Verification items for this drawing (mm, ordinates from the low corner). Round coordinates to 2 decimals unless told otherwise and drop trailing zeros. Order: outer loops, then holes, each group sorted by start corner. A loop starts at its lowest first (then second) coordinate and runs counter-clockwise, first axis right, second up. Notation, with made-up numbers: (-34.75, 40) -> (-5.75, 40) arc R23 ccw to (-5.75, 48) -> close; hole circle Ø10 at (28.25, -11). An arc over 180 degrees is marked (long way). Answer in a Markdown table with one row per item. Add a question column.
1. Sectioned sample at B-B, the plane z = 10. Record the boundary of the cut face in (x, y), then the cut area to 3 significant figures.
2. Depth check by flat-ended pin: P1, Ø4.5, axis at x = 60, z = 60, coming from the +Y side. Enter the tip coordinate at first touch or a pass-through.
3. Sectioned sample at A-A, the plane x = 60. Record the boundary of the cut face in (y, z).
4. Material ranges on L1, parallel to Z at x = 60, y = 6; L2, parallel to X at y = 3.5, z = 59; L3, parallel to Z at x = 9.5, y = 1, recorded low to high. Write a range as from..to.
5. Sectioned sample at C-C, the plane y = 7. Record the boundary of the cut face in (x, z).
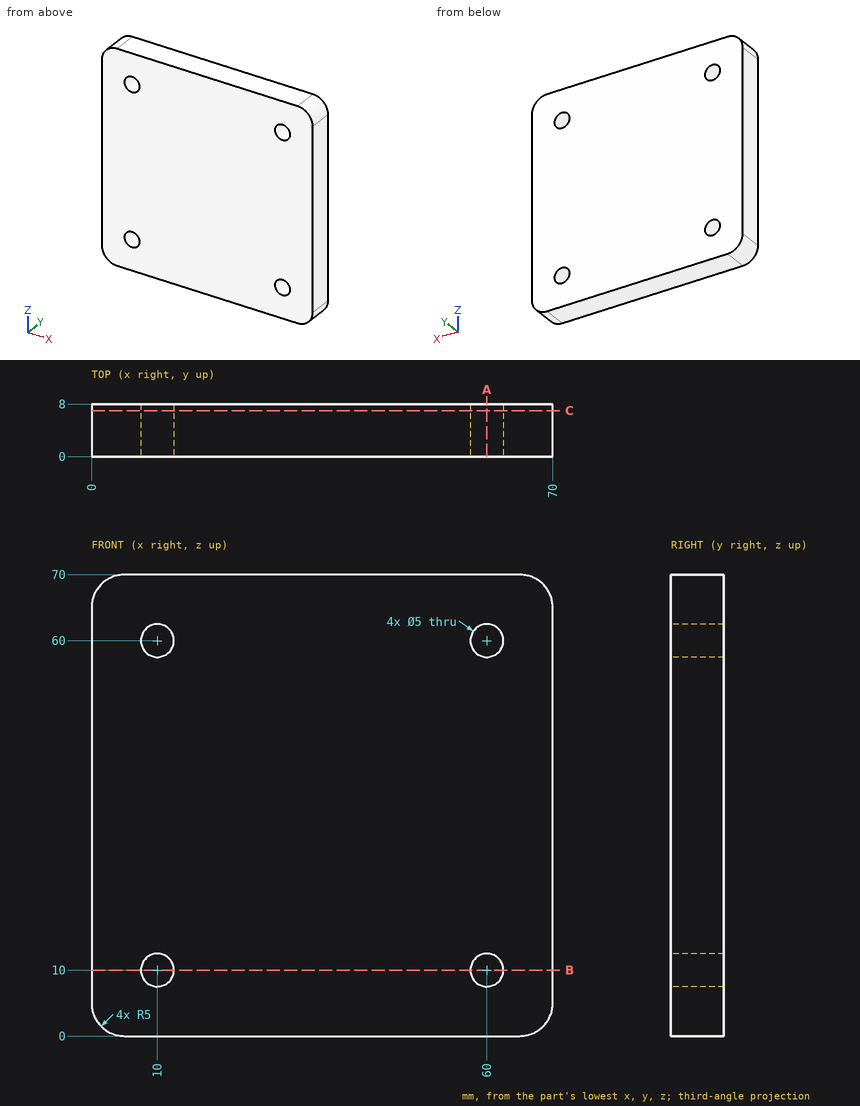
Answer key:
| question | item | result |
|---|---|---|
| 1 | outline | (0, 0) -> (7.5, 0) -> (7.5, 8) -> (0, 8) -> close; (12.5, 0) -> (57.5, 0) -> (57.5, 8) -> (12.5, 8) -> close; (62.5, 0) -> (70, 0) -> (70, 8) -> (62.5, 8) -> close |
| 1 | area | 480 mm² |
| 2 | P1 | passes through |
| 3 | outline | (0, 0) -> (8, 0) -> (8, 7.5) -> (0, 7.5) -> close; (0, 12.5) -> (8, 12.5) -> (8, 57.5) -> (0, 57.5) -> close; (0, 62.5) -> (8, 62.5) -> (8, 70) -> (0, 70) -> close |
| 4 | L1 | z = 0..7.5, 12.5..57.5, 62.5..70 |
| 4 | L2 | x = 0..7.71, 12.29..57.71, 62.29..70 |
| 4 | L3 | z = 0..7.55, 12.45..57.55, 62.45..70 |
| 5 | outline | (0, 5) arc R5 ccw to (5, 0) -> (65, 0) arc R5 ccw to (70, 5) -> (70, 65) arc R5 ccw to (65, 70) -> (5, 70) arc R5 ccw to (0, 65) -> close; hole circle Ø5 at (10, 10); hole circle Ø5 at (10, 60); hole circle Ø5 at (60, 10); hole circle Ø5 at (60, 60) |
